The listing builds one solid part. Answer for the finished solid, in the listing's coordinates (mm). Face numbers are marked on the shaded views. Give positions to 0.01 mm unless a question says otherwise; leave off trailing zeros. Order: outer loops, then holes, each group sorted by start corner. A loop starts at its lowest first (then second) coordinate and runs counter-clockwise, first axis right, second up. Notation, with made-up numbers: (67.25, 43.5) - (112.25, 43.5) arc R14 cw to (112.25, 68.5) - close; hole circle Ø2 at (-31.75, 43.5). An arc over 180 degrees is marked (long way). Write each question's results on one line, items separated by ' | '. Start each with the question number.
1. Section C-C (x = -182) is taken. Give the vertices of the cut face in (y, z), and give its area (3 significant figures).
2. Determine the mould class of the marked faces 1 and 2 for opening direction X: released by +X, released by -X, zero draft, split by the parting line, or undercut.
3. Section A-A (y = 146) is taken. Give the vertices of the cut face in (x, z), and give its area (3 significant figures).
4. Flat-ended cylindrical pins translate along their axes: pin 1 (2 mm diameter, centred on x = 257.5, z = 5, fed in from +Y); pin 2 (3.5 mm diameter, centred on y = 401, z = 2, fed in from +X); pin 3 (6 mm diameter, centred on x = -53.5, z = 4.5, fed in from -Y). Find the tip coordinate at first contact, or state that the pin passes through.
5. Section D-D (y = 349) is taken. Give the vertices of the cut face in (x, z), and give its area (3 significant figures).
6. Section B-B (z = 21) is taken. Give the vertices of the cut face in (x, y), and give its area (3 significant figures).
7. Find the intervals of material crossed by L1, parallel to X at y = 41.5, z = 23.5; L2, parallel to Y at x = -262.5, z = 19; L3, parallel to X at y = 42, z = 42.5, in increasing order.
from build123d import *

# Parameters (mm, degrees)
SKETCH1_R           = 16.5
SKETCH1_R_2         = 15
BOSS_EXTRUDE3_DEPTH = 7
SKETCH2_R           = 27.5
SKETCH2_R_2         = 16.5
BOSS_EXTRUDE4_DEPTH = 38
BOSS_EXTRUDE5_DEPTH = 7


with BuildPart() as part:
    # Sketch1 → Boss-Extrude3 (new body)
    with BuildSketch(Plane.XY):
        with BuildLine():
            Line((-322.811275448, 54.020092964), (-308.016991909, 51.544375984))
            ThreePointArc((-308.016991909, 51.544375984), (-297.979605272, 15.041649319), (-263.634141291, -0.882774953))
            Line((-263.634141291, -0.882774953), (-262.985194212, -0.878095462))
            ThreePointArc((-262.985194212, -0.878095462), (-234.213459723, 10.066916736), (-219.209238471, 36.945892575))
            ThreePointArc((-219.209238471, 36.945892575), (-5.54789332, 226.171081865), (222.17000985, 54.119057031))
            ThreePointArc((222.17000985, 54.119057031), (271.744200091, 2.083431527), (308.115870104, 64.070593748))
            Line((308.115870104, 64.070593748), (322.942948353, 66.658271071))
            ThreePointArc((322.942948353, 66.658271071), (72.802770658, 324.018256719), (-281.327086526, 382.296168148))
            ThreePointArc((-281.327086526, 382.296168148), (-317.291599122, 361.87304371), (-330.761322011, 322.769121357))
            Line((-330.761322011, 322.769121357), (-322.811275448, 54.020092964))
        make_face()
        with Locations((-263.634141291, 44.117225047)):
            Circle(SKETCH1_R, mode=Mode.SUBTRACT)
        with Locations((266.5683015, 46.784774614)):
            Circle(SKETCH1_R, mode=Mode.SUBTRACT)
        with Locations((-186.584414745, 266.470160007)):
            Circle(SKETCH1_R_2, mode=Mode.SUBTRACT)
        with Locations((-272.286901184, 324.498892702)):
            Circle(SKETCH1_R_2, mode=Mode.SUBTRACT)
    extrude(amount=BOSS_EXTRUDE3_DEPTH)

    # Sketch2 → Boss-Extrude4 (add)
    with BuildSketch(Plane.XY.offset(7)):
        with Locations((-263.634141291, 44.117225047)):
            Circle(SKETCH2_R)
        with Locations((-263.634141291, 44.117225047)):
            Circle(SKETCH2_R_2, mode=Mode.SUBTRACT)
        with Locations((266.5683015, 46.784774614)):
            Circle(SKETCH2_R)
        with Locations((266.5683015, 46.784774614)):
            Circle(SKETCH2_R_2, mode=Mode.SUBTRACT)
    extrude(amount=BOSS_EXTRUDE4_DEPTH)

    # Sketch3 → Boss-Extrude5 (add)
    with BuildSketch(Plane.XY.offset(7)):
        Polygon((-263.634141291, 408.541652183), (-263.634141291, 384.267252813), (-163.635450853, 388.029879984), (-163.635450853, 408.029879984), align=None)
        Polygon((-326.306060919, 172.160306647), (-346.306060919, 172.160306647), (-346.306060919, 72.160306647), (-323.347893363, 72.160306647), align=None)
        Polygon((244.528320181, 186.784774614), (312.652861422, 86.784774614), (330.829684073, 104.1400142), (274.528320181, 186.784774614), align=None)
    extrude(amount=-BOSS_EXTRUDE5_DEPTH)


solid = part.part
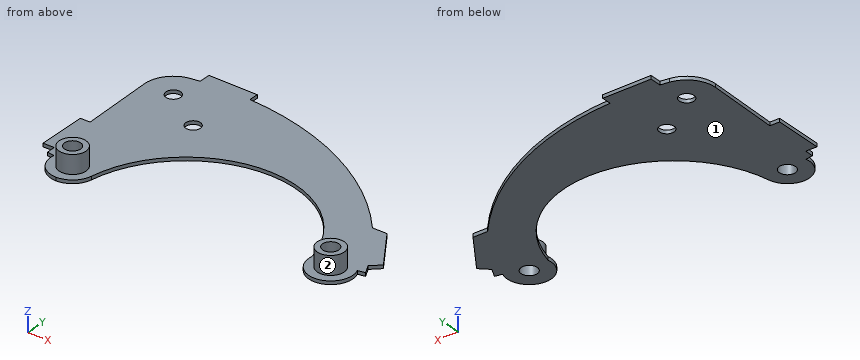
Reported:
1) outline: (129.33, 0) - (252.19, 0) - (252.19, 7) - (129.33, 7) - close; (280.75, 0) - (408.12, 0) - (408.12, 7) - (280.75, 7) - close | area: 1,750 mm²
2) face 1: zero draft | face 2: undercut
3) outline: (-346.31, 0) - (-169.26, 0) - (-169.26, 7) - (-346.31, 7) - close; (175.68, 0) - (302.31, 0) - (302.31, 7) - (175.68, 7) - close | area: 2,130 mm²
4) pin 1: y = 186.78 | pin 2: x = -163.64 | pin 3: y = 218.28
5) outline: (-325.41, 0) - (18.18, 0) - (18.18, 7) - (-325.41, 7) - close | area: 2,410 mm²
6) outline: circle Ø55 at (-263.63, 44.12); circle Ø55 at (266.57, 46.78); hole circle Ø33 at (-263.63, 44.12); hole circle Ø33 at (266.57, 46.78) | area: 3,040 mm²
7) L1: -291.01 to -279.93, -247.34 to -236.26, 239.58 to 250.94, 282.2 to 293.56 | L2: 16.64 to 27.66, 60.58 to 71.59 | L3: -291.05 to -280, -247.27 to -236.22, 239.49 to 250.78, 282.36 to 293.65
